Part model, mm, in its own coordinate system. A direction names the side the tool comes from. Coordinates: 2 decimals unless noted, no trailing zeros. Write each loop counter-clockwise with the first axis right and the second up, starting at its lowest first coordinate (ties: lowest second). Pieces come first, ordered by that corner, then holes. Notation, with made-up numbers: (-17, -12) -> (-3, -12) arc R24 cw to (-3, 20) -> close; hole circle Ø6 at (67, -12.5). An arc over 180 degrees is marked (long way). Write item = value, one per line. Start each with the question number.
Q1. Band-saw the part on A-A, the plane x = 15.5. List the corners of the cut face in (y, z).
Q2. Tool access for faces 4 (the flat face through (10, -50, 19)), 5 (the cylindrical face through (-0.57, -48.964, 12.175)), 6 (the flat face through (42.5, -47, 38)): list every direction of +Z, -Z, +X, -X, +Y, -Y with a clear straight run to the whole face (end or side of a thin tool).
Q3. Band-saw the part on D-D, the plane x = 44. List the corners of the cut face in (y, z).
Q4. Probe line 1 (X direction, y = -47.5, z = 5.25); line 2 (Y direction, x = 23.5, z = 4.25); line 3 (X direction, y = -48.25, z = 15). List the from-to ranges inside material, lowest first.
Q5. Band-saw the part on B-B, the plane z = 25. List the corners of the cut face in (x, y).
Q6. Pull direction Y, two halves, no side cores. Call faces 1 (the flat face through (10, -45, 19)), 2 (the cylindrical face through (47.57, -48.964, 37.825)), 3 (the flat face through (52.5, -48, 25)): released by +Y, released by -Y, zero draft, split by the parting line, or undercut.
Q7. Band-saw the part on C-C, the plane z = 44. List the corners of the cut face in (x, y).
Q8. Pin check, flat tips, straight feed: P1, Ø1.8, axis at x = 23.5, y = -47.5, coming from the +Z side; P2, Ø1.5, axis at y = -47, z = 37.5, coming from the -X side; P3, Ø1.8, axis at y = -47.5, z = 12.5, coming from the +X side. Stop position of each tip, or through.
from build123d import *

# Parameters (mm, degrees)
ESQUISSE1_W             = 58
ESQUISSE1_H             = 5
BOSS_EXTRU_1_DEPTH      = 50
ESQUISSE2_R             = 15
ENL_V_MAT_EXTRU_1_DEPTH = 6
ESQUISSE3_R             = 1.5
ENL_V_MAT_EXTRU_2_DEPTH = 10
ESQUISSE4_R             = 1.5
ENL_V_MAT_EXTRU_3_DEPTH = 10
ESQUISSE5_R             = 1.5
ENL_V_MAT_EXTRU_4_DEPTH = 51


with BuildPart() as part:
    # Esquisse1 → Boss.-Extru.1 (new body)
    with BuildSketch(Plane.XY):
        with Locations((23.5, -47.5)):
            Rectangle(ESQUISSE1_W, ESQUISSE1_H)
    extrude(amount=BOSS_EXTRU_1_DEPTH)

    # Esquisse2 → Enlèv. mat.-Extru.1 (cut, through all)
    with BuildSketch(Plane(origin=(0, -45, 0), x_dir=(-1, 0, 0), z_dir=(0, 1, 0))):
        with Locations((-24.5, 25)):
            Circle(ESQUISSE2_R)
    extrude(amount=-ENL_V_MAT_EXTRU_1_DEPTH, mode=Mode.SUBTRACT)

    # Esquisse3 → Enlèv. mat.-Extru.2 (cut)
    with BuildSketch(Plane.ZY.offset(5.5)):
        with Locations((12.5, -47.5)):
            Circle(ESQUISSE3_R)
        with Locations((37.5, -47.5)):
            Circle(ESQUISSE3_R)
    extrude(amount=-ENL_V_MAT_EXTRU_2_DEPTH, mode=Mode.SUBTRACT)

    # Esquisse4 → Enlèv. mat.-Extru.3 (cut)
    with BuildSketch(Plane(origin=(52.5, 0, 0), x_dir=(0, 0, -1), z_dir=(1, 0, 0))):
        with Locations((-37.5, -47.5)):
            Circle(ESQUISSE4_R)
        with Locations((-12.5, -47.5)):
            Circle(ESQUISSE4_R)
    extrude(amount=-ENL_V_MAT_EXTRU_3_DEPTH, mode=Mode.SUBTRACT)

    # Esquisse5 → Enlèv. mat.-Extru.4 (cut, through all)
    with BuildSketch(Plane.XY.offset(50)):
        with Locations((23.5, -47.5)):
            Circle(ESQUISSE5_R)
    extrude(amount=-ENL_V_MAT_EXTRU_4_DEPTH, mode=Mode.SUBTRACT)


solid = part.part
Ans:
q1.outline = (-50, 0) -> (-45, 0) -> (-45, 13) -> (-50, 13) -> close; (-50, 37) -> (-45, 37) -> (-45, 50) -> (-50, 50) -> close
q2.face_4 = +Z, -Z, +X, -X, -Y
q2.face_5 = -X
q2.face_6 = +X
q3.outline = (-50, 0) -> (-45, 0) -> (-45, 50) -> (-50, 50) -> close; hole circle Ø3 at (-47.5, 12.5); hole circle Ø3 at (-47.5, 37.5)
q4.line_1 = -5.5 to 22, 25 to 52.5
q4.line_2 = -50 to -49, -46 to -45
q4.line_3 = -5.5 to 13.32, 35.68 to 52.5
q5.outline = (-5.5, -50) -> (9.5, -50) -> (9.5, -45) -> (-5.5, -45) -> close; (39.5, -50) -> (52.5, -50) -> (52.5, -45) -> (39.5, -45) -> close
q6.face_1 = released by +Y
q6.face_2 = undercut
q6.face_3 = zero draft
q7.outline = (-5.5, -50) -> (52.5, -50) -> (52.5, -45) -> (-5.5, -45) -> close; hole circle Ø3 at (23.5, -47.5)
q8.P1 = through
q8.P2 = 4.5
q8.P3 = 42.5
